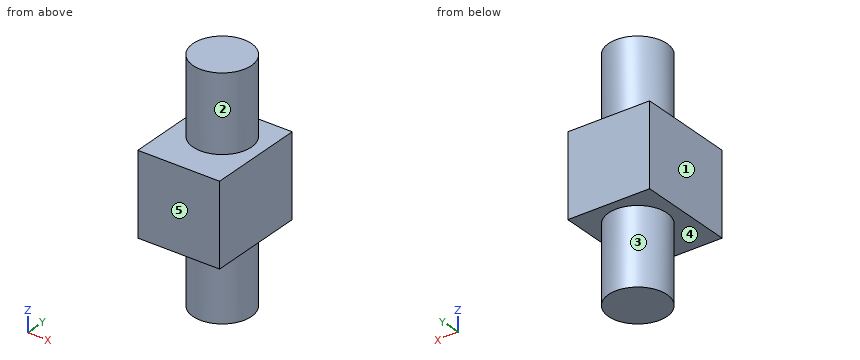
```python
from build123d import *

# Parameters (mm, degrees)
SKETCH1_W                = 42
SKETCH1_H                = 42
BOSS_EXTRUDE1_DEPTH      = 50
BOSS_EXTRUDE2_DEPTH      = 60
BOSS_EXTRUDE2_DEPTH_BACK = 60
SKETCH2_R                = 15


with BuildPart() as part:
    # Sketch1 → Boss-Extrude1 (new body)
    with BuildSketch(Plane(origin=(0, 0, 0), x_dir=(1, 0, 0), z_dir=(0, 1, 0))):
        Rectangle(SKETCH1_W, SKETCH1_H)
    extrude(amount=BOSS_EXTRUDE1_DEPTH)

    # Sketch2 → Boss-Extrude2 (add, two sides: drawn at the far end of the back side and taken through both)
    with BuildSketch(Plane.XY.offset(-BOSS_EXTRUDE2_DEPTH_BACK)):
        with Locations((0, 30)):
            Circle(SKETCH2_R)
    extrude(amount=BOSS_EXTRUDE2_DEPTH + BOSS_EXTRUDE2_DEPTH_BACK)


solid = part.part
```
Geometry: final body of the model. Coordinates: model frame, mm. Face numbers are marked on the shaded views. A direction names the side the tool comes from. Give positions to 0.01 mm unless a question says otherwise; leave off trailing zeros. Loops run counter-clockwise (first coordinate to the right, second up) from the corner with the lowest first, then second, coordinate; pieces in that order, holes last. Notation, with made-up numbers: (-12.75, 52) - (11.25, 52) arc R10 ccw to (11.25, 59) - close; hole circle Ø6 at (69, 69.5). An arc over 180 degrees is marked (long way). Answer as CSV lines item,"result". Start each with the question number.
(1) Section query A-A (x = 0). Output: boundary loops of the cut face in (y, z), and give its area (3 significant figures).
(2) Section query C-C (z = -52). Output: boundary loops of the cut face in (x, y).
(3) Ray query, line 1 along Z through (x, y) = (-16.5, 36); line 2 along Y through (x, z) = (-8, 50); line 3 along Y through (x, z) = (13, -35). Return the intervals inside material, ascending. Write a range as [from, to].
(4) Section query D-D (y = 12). Output: boundary loops of the cut face in (x, z), and give its area (3 significant figures).
(5) Reachability of the marked faces 1 and 2 from +Z, -Z, +X, -X, +Y, -Y: full face, straight path, thin tool, end or side. Return the list, or none.
(6) Mould query, pull axis Y, two halves, no side actions, for the marked faces 3, 4 and 5. Classes: +Y half, -Y half, draft (parallel to the pull), parting line (faces both ways), or undercut.
(7) Pin query (flat end, axial travel): P1, Ø8, axis at x = -14.5, y = 11, coming from the -Z side. Return the tip coordinate at first contact, or that it passes through.
(8) Section query B-B (y = 30). Output: boundary loops of the cut face in (x, z).
Worked answers:
1,outline,"(0, -21) - (15, -21) - (15, -60) - (45, -60) - (45, -21) - (50, -21) - (50, 21) - (45, 21) - (45, 60) - (15, 60) - (15, 21) - (0, 21) - close"
1,area,"4,440 mm^2"
2,outline,"circle Ø30 at (0, 30)"
3,line 1,"z = [-21, 21]"
3,line 2,"y = [17.31, 42.69]"
3,line 3,"y = [22.52, 37.48]"
4,outline,"(-21, -21) - (21, -21) - (21, 21) - (-21, 21) - close"
4,area,"1,760 mm^2"
5,face 1,"+Z, -Z, -X, +Y, -Y"
5,face 2,"+Z"
6,face 3,"parting line"
6,face 4,"draft"
6,face 5,"-Y half"
7,P1,"stops at z = -21"
8,outline,"(-21, -21) - (-15, -21) - (-15, -60) - (15, -60) - (15, -21) - (21, -21) - (21, 21) - (15, 21) - (15, 60) - (-15, 60) - (-15, 21) - (-21, 21) - close"
